Could you check a few things on this model? Use its own coordinates, in mm. A direction names the side the tool comes from. Give positions to 0.01 mm unless a question says otherwise; leave off trailing zeros. Loops run counter-clockwise (first coordinate to the right, second up) from the corner with the lowest first, then second, coordinate; pieces in that order, holes last. Notation, with made-up numbers: M 18.5,16 L 30.5,16 A20 cw 30.5,21 Z; hole C -9.75,77 d2. An arc over 180 degrees is marked long. Answer in a Markdown table with one row per item. Add a question column.
1. I need wall thicknesses on line 1 along X through (y, z) = (-0.5, -17); line 2 along X through (y, z) = (-3.5, -10); line 3 along Z through (x, y) = (-80.5, -0.5). Which ranges of each line are inside material? Lowest first, please. Write a range as from..to.
2. If we section it at A-A on x = -183.5: List the corners of the cut face in (y, z) for me, then the cut area to 3 significant figures.
3. Thinking about a two-plate mould opening in X: for faces 3 (the flat face through (-254, 0, 0)), 4 (the cylindrical face through (-128.78, -1.38, 6.2)), 5 (the flat face through (0, 0, 0)), which applies, released by +X, released by -X, zero draft, split by the parting line, or undercut?
4. If we section it at B-B on z = 2.5: List the corners of the cut face in (x, y) for me.
5. I'm going to push flat-ended pins straight in: pin 1 Ø2.5 at (x, y) = (-222.19, 0) entering from -Z; pin 2 Ø3.5 at (x, y) = (-31.69, 0) entering from -Z; pin 3 Ø2 at (x, y) = (-32.5, -3.5) entering from +Z; pin 4 Ø4 at (x, y) = (-210.5, -2.5) entering from -Z. Where does each tip first touch, or does it pass through?
6. Which directions (+Z, -Z, +X, -X, +Y, -Y) give clear straight access to the entire face, cutting with the end or side of a thin tool? Please do faces 1 (the flat face through (-30, -1, -31.75)), 2 (the cylindrical face through (-38.038, -0.279, -19.625)).
```python
from build123d import *

# Parameters (mm, degrees)
F1_R     = 6.35
F3_R     = 6.35
F6_D     = 3.175
F6_DEPTH = 12.7
F6_TIP   = 0.9538662327


with BuildPart() as f2:
    # F2: sweep along a path in F0
    with BuildLine(Plane.XZ) as f2_path:
        Line((0, 0), (-254, 0))
    # F1 (on Right) → F2 (sweep)
    with BuildSketch(Plane.YZ):
        Circle(F1_R)
    sweep(path=f2_path.line)

    # F4: sweep along a path in F0
    with BuildLine(Plane.XZ) as f4_path:
        Line((-222.25, 0), (-222.25, -31.75))
    # F3 (on Top) → F4 (sweep)
    with BuildSketch(Plane.XY):
        with Locations((-222.1939712763, 0)):
            Circle(F3_R)
        with Locations((-31.6939712763, 0)):
            Circle(F3_R)
    sweep(path=f4_path.line)

    # F6
    with Locations(Plane(origin=(0, 0, -31.75), x_dir=(1, 0, 0), z_dir=(0, 0, -1))):
        with Locations((-222.1939712763, 0), (-31.6939712763, 0)):
            Hole(F6_D / 2, depth=F6_DEPTH)
            with Locations((0, 0, -(F6_DEPTH + F6_TIP / 2))):  # 118° drill point
                Cone(0, F6_D / 2, F6_TIP, mode=Mode.SUBTRACT)


solid = f2.part
```
Results:
| question | item | result |
|---|---|---|
| 1 | line 1 | -228.52..-215.86, -38.02..-25.36 |
| 1 | line 2 | -227.49..-216.9, -36.99..-26.4 |
| 1 | line 3 | -6.33..6.33 |
| 2 | outline | C 0,0 d12.7 |
| 2 | area | 127 mm2 |
| 3 | face 3 | released by -X |
| 3 | face 4 | undercut |
| 3 | face 5 | released by +X |
| 4 | outline | M -254,-5.84 L 0,-5.84 L 0,5.84 L -254,5.84 Z |
| 5 | pin 1 | z = -18.85 |
| 5 | pin 2 | z = -31.75 |
| 5 | pin 3 | z = 5.84 |
| 5 | pin 4 | z = -6.33 |
| 6 | face 1 | -Z, +X, -X, +Y, -Y |
| 6 | face 2 | -Z |
